Can you work these out from the model? Positions are in its coordinate system, mm. A direction names the side the tool comes from. Coordinates: 2 decimals unless noted, no trailing zeros. Order: outer loops, then holes, each group sorted by start corner. A loop starts at its lowest first (then second) coordinate and runs counter-clockwise, first axis right, second up. Notation, with made-up numbers: (-18, 4) -> (-1, 4) arc R13 ccw to (-1, 16) -> close; hole circle Ø3 at (41.5, 3.5). An arc over 180 degrees is marked (long way). Write item = value, one per line. Start each with the question number.
from build123d import *

# Parameters (mm, degrees)
SKETCH1_W           = 30.2180244
SKETCH1_H           = 30.2180244
SKETCH1_R           = 9.3599
SKETCH1_R_2         = 1.7018
BOSS_EXTRUDE1_DEPTH = 0.79375
SKETCH2_W           = 30.2180244
SKETCH2_H           = 33.02
BOSS_EXTRUDE2_DEPTH = 0.79375
BOSS_EXTRUDE3_DEPTH = 0.79375
BOSS_EXTRUDE4_DEPTH = 0.79375
CUT_EXTRUDE1_DEPTH  = 55.453462241


with BuildPart() as part:
    # Sketch1 → Boss-Extrude1 (new body)
    with BuildSketch(Plane(origin=(0, 0, 0), x_dir=(1, 0, 0), z_dir=(0, 1, 0))):
        with Locations((15.1090122, -15.1090122)):
            Rectangle(SKETCH1_W, SKETCH1_H)
        with Locations(Location((15.1090122, -15.1090122, 0), (0, 0, 270))):
            Circle(SKETCH1_R, mode=Mode.SUBTRACT)
        with Locations(Location((2.7900122, -2.7900122, 0), (0, 0, 270))):
            Circle(SKETCH1_R_2, mode=Mode.SUBTRACT)
        with Locations(Location((27.4280122, -2.7900122, 0), (0, 0, 270))):
            Circle(SKETCH1_R_2, mode=Mode.SUBTRACT)
        with Locations(Location((27.4280122, -27.4280122, 0), (0, 0, 270))):
            Circle(SKETCH1_R_2, mode=Mode.SUBTRACT)
        with Locations(Location((2.7900122, -27.4280122, 0), (0, 0, 270))):
            Circle(SKETCH1_R_2, mode=Mode.SUBTRACT)
    extrude(amount=BOSS_EXTRUDE1_DEPTH)

    # Sketch2 → Boss-Extrude2 (add)
    with BuildSketch(Plane.XY.offset(30.2180244)):
        with Locations((15.1090122, 16.51)):
            Rectangle(SKETCH2_W, SKETCH2_H)
    extrude(amount=BOSS_EXTRUDE2_DEPTH)

    # Sketch3 → Boss-Extrude3 (add)
    with BuildSketch(Plane(origin=(30.2180244, 0, 0), x_dir=(0, 0, -1), z_dir=(1, 0, 0))):
        Polygon((-25.1380244, 0.79375), (-30.2180244, 5.87375), (-30.2180244, 33.02), (-31.0117744, 33.02), (-31.0117744, 0), (0, 0), (0, 0.79375), align=None)
    extrude(amount=BOSS_EXTRUDE3_DEPTH)

    # Sketch4 → Boss-Extrude4 (add)
    with BuildSketch(Plane.ZY):
        Polygon((25.1380244, 0.79375), (30.2180244, 5.87375), (30.2180244, 33.02), (31.0117744, 33.02), (31.0117744, 0), (0, 0), (0, 0.79375), align=None)
    extrude(amount=BOSS_EXTRUDE4_DEPTH)

    # Sketch5 → Cut-Extrude1 (cut, through all)
    with BuildSketch(Plane(origin=(0, 0, 30.2180244), x_dir=(-1, 0, 0), z_dir=(0, 0, -1))):
        with BuildLine():
            Line((-4.147269761, 4.395528514), (-4.147269761, 27.509830099))
            ThreePointArc((-4.147269761, 27.509830099), (-2.8177744, 28.83932546), (-1.488279039, 27.509830099))
            Line((-1.488279039, 27.509830099), (-1.488279039, 4.395528514))
            ThreePointArc((-1.488279039, 4.395528514), (-2.8177744, 3.066033153), (-4.147269761, 4.395528514))
        make_face()
        with BuildLine():
            Line((-28.785269761, 4.395528514), (-28.785269761, 27.509830099))
            ThreePointArc((-28.785269761, 27.509830099), (-27.4557744, 28.83932546), (-26.126279039, 27.509830099))
            Line((-26.126279039, 27.509830099), (-26.126279039, 4.395528514))
            ThreePointArc((-26.126279039, 4.395528514), (-27.4557744, 3.066033153), (-28.785269761, 4.395528514))
        make_face()
    extrude(amount=-CUT_EXTRUDE1_DEPTH, mode=Mode.SUBTRACT)


solid = part.part
(1) If I drill on L1, parallel to Z at x = 18.5, y = 9.5; L2, parallel to Y at x = 24, z = 4, over which ranges is the centre line in solid material (lowest first)? Write a range as from..to.
(2) For P1, Ø16, axis at x = 7.5, y = 12, coming from the -Z side, with a flat end and sliding along its axis, tell me the tip position at first contact or that it passes through.
(3) Thinking about a two-plate mould opening in Z: for faces 4 (the face through (15, 17, 30.218)), 5 (the face through (1.13, 0.39, 2.42)), 6 (the face through (22, 0, 23)), which applies, +Z half, -Z half, draft (parallel to the pull), parting line (faces both ways), or undercut?
(4) Imagine slicing it at B-B (z = 18). Write out the boundary of the cut face in (x, y), plus the area to 3 significant figures.
(5) For faces 1 (the face through (0, 2, 29)), 2 (the face through (28.578, 0.391, 26.174)), 3 (the face through (27.427, 3.066, 30.609)), which set-ups out of +Z, -Z, +X, -X, +Y, -Y let a thin tool reach every point of the face, with its end or its side?
(6) Imagine slicing it at A-A (y = 14.5). Write out the boundary of the cut face in (x, z), plus the area to 3 significant figures.
(7) Imagine slicing it at C-C (x = 11.5). Write out the boundary of the cut face in (y, z), plus the area to 3 significant figures.
(8) Imagine slicing it at D-D (x = 28). Write out the boundary of the cut face in (y, z), plus the area to 3 significant figures.
Result set:
q1.L1 = 30.22..31.01
q1.L2 = 0..0.79
q2.P1 = 30.22
q3.face_4 = -Z half
q3.face_5 = undercut
q3.face_6 = draft
q4.outline = (-0.79, 0) -> (6.21, 0) -> (6.21, 0.79) -> (-0.79, 0.79) -> close; (24.01, 0) -> (31.01, 0) -> (31.01, 0.79) -> (24.01, 0.79) -> close
q4.area = 11.1 mm2
q5.face_1 = -Z, +Y
q5.face_2 = +Y, -Y
q5.face_3 = +Z, -Z
q6.outline = (-0.79, 30.22) -> (1.49, 30.22) -> (1.49, 31.01) -> (-0.79, 31.01) -> close; (4.15, 30.22) -> (26.13, 30.22) -> (26.13, 31.01) -> (4.15, 31.01) -> close; (28.79, 30.22) -> (31.01, 30.22) -> (31.01, 31.01) -> (28.79, 31.01) -> close
q6.area = 21.0 mm2
q7.outline = (0, 0) -> (0.79, 0) -> (0.79, 6.47) -> (0, 6.47) -> close; (0, 23.75) -> (0.79, 23.75) -> (0.79, 30.22) -> (33.02, 30.22) -> (33.02, 31.01) -> (0, 31.01) -> close
q7.area = 36.5 mm2
q8.outline = (0, 0) -> (0.79, 0) -> (0.79, 1.19) -> (0, 1.19) -> close; (0, 4.39) -> (0.79, 4.39) -> (0.79, 25.83) -> (0, 25.83) -> close; (0, 29.03) -> (0.79, 29.03) -> (0.79, 30.22) -> (3.18, 30.22) -> (3.18, 31.01) -> (0, 31.01) -> close; (28.72, 30.22) -> (33.02, 30.22) -> (33.02, 31.01) -> (28.72, 31.01) -> close
q8.area = 24.8 mm2
